from build123d import *

# Parameters (mm, degrees)
SKETCH1_R           = 18.5
BOSS_EXTRUDE1_DEPTH = 33
SKETCH4_R           = 16.5
CUT_EXTRUDE3_DEPTH  = 12.6
SKETCH5_W           = 20
SKETCH5_H           = 49.349350968
CUT_EXTRUDE4_DEPTH  = 20.4
SKETCH7_W           = 56.502792025
SKETCH7_H           = 7.03676062
CUT_EXTRUDE5_DEPTH  = 6.8


with BuildPart() as part:
    # Sketch1 → Boss-Extrude1 (new body)
    with BuildSketch(Plane(origin=(0, 0, 0), x_dir=(1, 0, 0), z_dir=(0, 1, 0))):
        with Locations(Location((0, 0, 0), (0, 0, 270))):
            Circle(SKETCH1_R)
    extrude(amount=BOSS_EXTRUDE1_DEPTH)

    # Sketch4 → Cut-Extrude3 (cut)
    with BuildSketch(Plane.XZ):
        with Locations(Location((0, 0, 0), (0, 0, 270))):
            Circle(SKETCH4_R)
    extrude(amount=-CUT_EXTRUDE3_DEPTH, mode=Mode.SUBTRACT)

    # Sketch5 → Cut-Extrude4 (cut)
    with BuildSketch(Plane(origin=(0, 33, 0), x_dir=(1, 0, 0), z_dir=(0, 1, 0))):
        Rectangle(SKETCH5_W, SKETCH5_H)
    extrude(amount=-CUT_EXTRUDE4_DEPTH, mode=Mode.SUBTRACT)

    # Sketch7 → Cut-Extrude5 (cut, symmetric)
    with BuildSketch(Plane(origin=(0, 0, 0), x_dir=(0.9821726027310876, 0, 0.1879813247225403), z_dir=(-0.1879813247225403, 0, 0.9821726027310876))):
        with Locations((-1.059105512, 31.21838031)):
            Rectangle(SKETCH7_W, SKETCH7_H)
    extrude(amount=CUT_EXTRUDE5_DEPTH, both=True, mode=Mode.SUBTRACT)


solid = part.part
Can you work these out from the model? Positions are in its coordinate system, mm. A direction names the side the tool comes from. Give positions to 0.01 mm unless a question says otherwise; leave off trailing zeros. Order: outer loops, then holes, each group sorted by start corner. A loop starts at its lowest first (then second) coordinate and runs counter-clockwise, first axis right, second up. Notation, with made-up numbers: M 3,-22.5 L 44,-22.5 A17 cw 44,7.5 Z; hole C 59.25,70.5 d2. An arc over 180 degrees is marked long. Use one line per item in the form item = value. Start each with the question number.
Item 1: If we section it at D-D (y = 23.5): Write out the boundary of the cut face in (x, z).
Item 2: Will these pins go through, and if not, where does the flat tip stop? pin 1 Ø10 at (x, z) = (-13.5, -4) entering from +Y; pin 2 Ø3 at (y, z) = (14.5, 9.5) entering from +X; pin 3 Ø2 at (x, z) = (12.5, -2.5) entering from -Y.
Item 3: For faces 5 (the flat face through (0, 0, -17)), 6 (the flat face through (0, 12.6, -17)), 7 (the flat face through (-12, 12.6, 0)), 8 (the flat face through (-14.145, 30.387, 4.216)), 9 (the flat face through (14.03, 30.39, -4.24)), which set-ups out of +Z, -Z, +X, -X, +Y, -Y let a thin tool reach every point of the face, with its end or its side?
Item 4: If I drill on line 1 along X through (y, z) = (5, 0); line 2 along Y through (x, z) = (13, 6.5), over which ranges is the centre line in solid material (lowest first)?
Item 5: If we section it at B-B (y = 31.5): Write out the boundary of the cut face in (x, z).
Item 6: We'd pull the mould along Z, two halves only. Please class faces 1 (the flat face through (13, 33, -8)), 2 (the flat face through (13, 27.7, 3)), 3 (the flat face through (12.771, 30.387, 9.368)), 4 (the cylindrical face through (-11.26, 12.6, -14.68)): +Z half, -Z half, draft (parallel to the pull), parting line (faces both ways), or undercut.
Item 7: If we section it at A-A (z = 0): Write out the boundary of the cut face in (x, y).
Item 8: If we section it at C-C (x = 0): Write out the boundary of the cut face in (y, z).
Outcome:
q1.outline = M -10,-15.56 L -10,15.56 A18.5 ccw Z; M 10,-15.56 A18.5 ccw 10,15.56 Z
q2.pin_1 = 27.7
q2.pin_2 = 16.68
q2.pin_3 = 12.6
q3.face_5 = +Z, -Z, +X, -X, -Y
q3.face_6 = +Z, -Z, +Y
q3.face_7 = -Y
q3.face_8 = +X, +Y
q3.face_9 = -X, +Y
q4.line_1 = -18.5 to -16.5, 16.5 to 18.5
q4.line_2 = 12.6 to 27.7
q5.outline = M -18.18,3.44 L -10,5.01 L -10,15.56 A18.5 ccw Z; M -15.62,-9.91 A18.5 ccw -10,-15.56 L -10,-8.84 Z; M 10,-15.56 A18.5 ccw 18.18,-3.44 L 10,-5.01 Z; M 10,8.84 L 15.62,9.91 A18.5 ccw 10,15.56 Z
q6.face_1 = draft
q6.face_2 = undercut
q6.face_3 = undercut
q6.face_4 = parting line
q7.outline = M -18.5,0 L -16.5,0 L -16.5,12.6 L -10,12.6 L -10,27.7 L -18.5,27.7 Z; M 10,12.6 L 16.5,12.6 L 16.5,0 L 18.5,0 L 18.5,27.7 L 10,27.7 Z
q8.outline = M 0,-18.5 L 12.6,-18.5 L 12.6,-16.5 L 0,-16.5 Z; M 0,16.5 L 12.6,16.5 L 12.6,18.5 L 0,18.5 Z
